Here's how the part is built. I have some questions about the finished solid (model axes, mm). Face numbers are marked on the shaded views. A direction names the side the tool comes from. Round coordinates to 2 decimals unless told otherwise and drop trailing zeros. Order: outer loops, then holes, each group sorted by start corner. A loop starts at its lowest first (then second) coordinate and runs counter-clockwise, first axis right, second up. Notation, with made-up numbers: (77, 88.5) -> (113, 88.5) arc R34 cw to (113, 119.5) -> close; hole circle Ø4 at (-31.5, 29.5). An arc over 180 degrees is marked (long way). Answer in a Markdown table with one row per item.
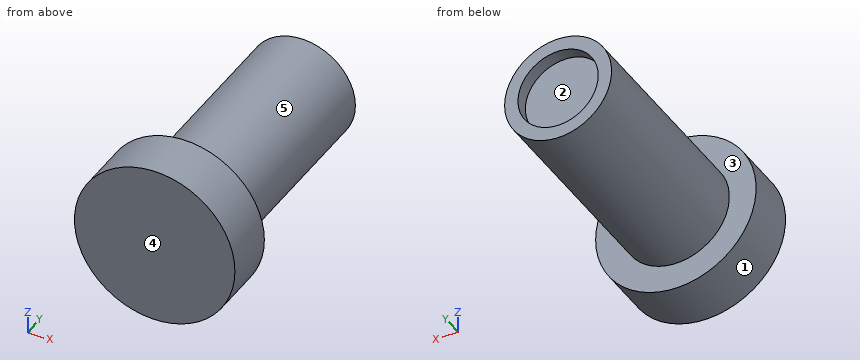
```python
from build123d import *

# Parameters (mm, degrees)
F0_R     = 6.35
F1_DEPTH = 25.4
F2_R     = 4.7625
F3_DEPTH = 1.5875
F4_R     = 9.525
F5_DEPTH = 6.35


with BuildPart() as f1:
    # F0 (on Front) → F1 (new body)
    with BuildSketch(Plane.XZ):
        Circle(F0_R)
    extrude(amount=F1_DEPTH)

    # F2 (on face) → F3 (cut)
    with BuildSketch(Plane(origin=(0, 0, 0), x_dir=(-1, 0, 0), z_dir=(0, 1, 0))):
        Circle(F2_R)
    extrude(amount=-F3_DEPTH, mode=Mode.SUBTRACT)

    # F4 (on face) → F5 (join)
    with BuildSketch(Plane.XZ.offset(25.4)):
        Circle(F4_R)
    extrude(amount=F5_DEPTH)


solid = f1.part
```
1. Suppose I cut it at C-C on y = -10. Write out the boundary of the cut face in (x, z).
Numbers:
| item | result |
|---|---|
| outline | circle Ø12.7 at (0, 0) |
2. For the marked faces 4 and 5, which set-ups out of +Z, -Z, +X, -X, +Y, -Y let a thin tool reach every point of the face, with its end or its side?
Numbers:
| item | result |
|---|---|
| face 4 | +Z, -Z, +X, -X, -Y |
| face 5 | +Y |
3. For pin 1 Ø4 at (x, y) = (1, -14) entering from -Z; pin 2 Ø6 at (y, z) = (-26, 6) entering from -X; pin 3 Ø4 at (x, y) = (0.5, -17) entering from +Z, each with a flat end and sliding along its axis, tell me the tip position at first contact or that it passes through.
Numbers:
| item | result |
|---|---|
| pin 1 | stops at z = -6.35 |
| pin 2 | stops at x = -9.04 |
| pin 3 | stops at z = 6.35 |
4. We'd pull the mould along Z, two halves only. Please class the marked faces 1, 2 and 3: released by +Z, released by -Z, zero draft, split by the parting line, or undercut.
Numbers:
| item | result |
|---|---|
| face 1 | split by the parting line |
| face 2 | undercut |
| face 3 | zero draft |
5. Please list where these lines run through material, in increasing order: line 1 along Z through (x, y) = (0, -1.2); line 2 along Y through (x, z) = (3.25, 3); line 3 along X through (y, z) = (-0.5, 1.75).
Numbers:
| item | result |
|---|---|
| line 1 | z = -6.35 to -4.76, 4.76 to 6.35 |
| line 2 | y = -31.75 to -1.59 |
| line 3 | x = -6.1 to -4.43, 4.43 to 6.1 |
6. Suppose I cut it at D-D on y = -29. Write out the boundary of the cut face in (x, z) (3 decimals), then the cut area to 3 significant figures.
Numbers:
| item | result |
|---|---|
| outline | circle Ø19.05 at (0, 0) |
| area | 285 mm2 |
